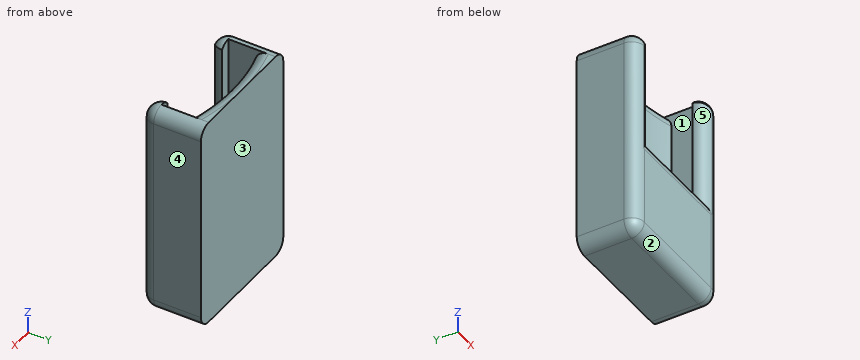
```python
from build123d import *

# Parameters (mm, degrees)
F0_W         = 53
F0_H         = 23.8
F0_W_2       = 43
F0_H_2       = 13.8
F1_DEPTH     = 80
F2_DEPTH     = 5
F3_W         = 35
F3_H         = 44
F4_DEPTH     = 25
F5_T1_DEPTH  = 78
F5_T3_DEPTH  = 110
F5_T5_DEPTH  = 35
F5_T7_DEPTH  = 56.5
F5_T13_DEPTH = 69
F5_T17_DEPTH = 47.5
F5_T24_DEPTH = 47.5
F5_T28_DEPTH = 69
F6_T1_DEPTH  = 31.3
F6_S5_W      = 5
F6_S5_H      = 5
F6_T6_DEPTH  = 5
F6_S11_W     = 5
F6_S11_H     = 5
F6_T12_DEPTH = 5
F7_R         = 4.99999
F9_DEPTH     = 80
F10_T4_ANGLE = 50.0121835392


# Not quite as in the source:
# - a fillet or chamfer that OpenCascade refuses, or shapes differently, is made with other operations: its cross-section is extruded or revolved along the edge and cut away or added
# - a fillet or chamfer is up to 0.001 mm smaller than in the source, because OpenCascade refuses the exact size


with BuildPart() as f1:
    # F0 (on Top) → F1 (new body)
    with BuildSketch(Plane.XY):
        with Locations((-2.25, 0.0045082584)):
            Rectangle(F0_W, F0_H)
        with Locations((-2.25, 0.0045082584)):
            Rectangle(F0_W_2, F0_H_2, mode=Mode.SUBTRACT)
    extrude(amount=F1_DEPTH)

    # F0 (on Top) → F2 (join)
    with BuildSketch(Plane.XY):
        with Locations((-2.25, 0.0045082584)):
            Rectangle(F0_W, F0_H)
        with Locations((-2.25, 0.0045082584)):
            Rectangle(F0_W_2, F0_H_2, mode=Mode.SUBTRACT)
        with Locations((-2.25, 0.0045082584)):
            Rectangle(F0_W_2, F0_H_2)
    extrude(amount=-F2_DEPTH)

    # F3 (on face) → F4 (cut)
    with BuildSketch(Plane(origin=(0, -6.8954917416, 0), x_dir=(-1, 0, 0), z_dir=(0, 1, 0))):
        with Locations((2.25, 58)):
            Rectangle(F3_W, F3_H)
    extrude(amount=-F4_DEPTH, mode=Mode.SUBTRACT)

    # F5: fillet of radius 5 on 6 edges, made by hand

    # F5_s2 → F5_t1 (cut)
    with BuildSketch(Plane.YZ.offset(-41.25)):
        with BuildLine():
            ThreePointArc((-11.8954917416, 0), (-10.4310256475, -3.5355339059), (-6.8954917416, -5))
            Line((-6.8954917416, -5), (-11.8954917416, -5))
            Line((-11.8954917416, -5), (-11.8954917416, 0))
        make_face()
    extrude(amount=F5_T1_DEPTH, mode=Mode.SUBTRACT)

    # F5_s4 → F5_t3 (cut)
    with BuildSketch(Plane.XY.offset(-17.5)):
        with BuildLine():
            ThreePointArc((-23.75, -11.8954917416), (-27.2855339059, -10.4310256475), (-28.75, -6.8954917416))
            Line((-28.75, -6.8954917416), (-28.75, -11.8954917416))
            Line((-28.75, -11.8954917416), (-23.75, -11.8954917416))
        make_face()
        with BuildLine():
            ThreePointArc((24.25, -6.8954917416), (22.7855339059, -10.4310256475), (19.25, -11.8954917416))
            Line((19.25, -11.8954917416), (24.25, -11.8954917416))
            Line((24.25, -11.8954917416), (24.25, -6.8954917416))
        make_face()
    extrude(amount=F5_T3_DEPTH, mode=Mode.SUBTRACT)

    # F5_s6 → F5_t5 (cut)
    with BuildSketch(Plane.YZ.offset(-19.75)):
        with BuildLine():
            ThreePointArc((-11.8954917416, 31), (-10.4310256475, 34.5355339059), (-6.8954917416, 36))
            Line((-6.8954917416, 36), (-11.8954917416, 36))
            Line((-11.8954917416, 36), (-11.8954917416, 31))
        make_face()
    extrude(amount=F5_T5_DEPTH, mode=Mode.SUBTRACT)

    # F5_s8 → F5_t7 (cut)
    with BuildSketch(Plane.XY.offset(36)):
        with BuildLine():
            ThreePointArc((-24.75, -11.8954917416), (-21.2144660941, -10.4310256475), (-19.75, -6.8954917416))
            Line((-19.75, -6.8954917416), (-19.75, -11.8954917416))
            Line((-19.75, -11.8954917416), (-24.75, -11.8954917416))
        make_face()
        with BuildLine():
            ThreePointArc((20.25, -11.8954917416), (16.7144660941, -10.4310256475), (15.25, -6.8954917416))
            Line((15.25, -6.8954917416), (15.25, -11.8954917416))
            Line((15.25, -11.8954917416), (20.25, -11.8954917416))
        make_face()
    extrude(amount=F5_T7_DEPTH, mode=Mode.SUBTRACT)


with BuildPart() as f5_tool11:
    # F5_s12 → F5_t13 (new body)
    with BuildSketch(Plane.XY.offset(92.5)):
        with BuildLine():
            ThreePointArc((20.25, -11.8954917416), (16.7144660941, -10.4310256475), (15.25, -6.8954917416))
            Line((15.25, -6.8954917416), (15.25, -11.8954917416))
            Line((15.25, -11.8954917416), (20.25, -11.8954917416))
        make_face()
    extrude(amount=-F5_T13_DEPTH)

    split(bisect_by=Plane.XY.offset(36), keep=Keep.BOTTOM)


with BuildPart() as f5_tool15:
    # F5_s16 → F5_t17 (new body)
    with BuildSketch(Plane.YZ.offset(27.75)):
        with BuildLine():
            ThreePointArc((-11.8954917416, 31), (-10.4310256475, 34.5355339059), (-6.8954917416, 36))
            Line((-6.8954917416, 36), (-11.8954917416, 36))
            Line((-11.8954917416, 36), (-11.8954917416, 31))
        make_face()
    extrude(amount=-F5_T17_DEPTH)

    split(bisect_by=Plane.YZ.offset(15.25), keep=Keep.TOP)


with BuildPart() as f5_tool11_1:
    add(f5_tool11.part)

    # F5_t19: intersect F5_tool15
    add(f5_tool15.part, mode=Mode.INTERSECT)


with BuildPart() as f1_1:
    add(f1.part)

    # F5_t9: cut F5_tool11
    add(f5_tool11_1.part, mode=Mode.SUBTRACT)


with BuildPart() as f5_tool22:
    # F5_s23 → F5_t24 (new body)
    with BuildSketch(Plane.YZ.offset(15.25)):
        with BuildLine():
            ThreePointArc((-11.8954917416, 31), (-10.4310256475, 34.5355339059), (-6.8954917416, 36))
            Line((-6.8954917416, 36), (-11.8954917416, 36))
            Line((-11.8954917416, 36), (-11.8954917416, 31))
        make_face()
    extrude(amount=-F5_T24_DEPTH)

    split(bisect_by=Plane.YZ.offset(-19.75), keep=Keep.BOTTOM)


with BuildPart() as f5_tool26:
    # F5_s27 → F5_t28 (new body)
    with BuildSketch(Plane.XY.offset(23.5)):
        with BuildLine():
            ThreePointArc((-24.75, -11.8954917416), (-21.2144660941, -10.4310256475), (-19.75, -6.8954917416))
            Line((-19.75, -6.8954917416), (-19.75, -11.8954917416))
            Line((-19.75, -11.8954917416), (-24.75, -11.8954917416))
        make_face()
    extrude(amount=F5_T28_DEPTH)

    split(bisect_by=Plane.XY.offset(36), keep=Keep.BOTTOM)


with BuildPart() as f5_tool22_1:
    add(f5_tool22.part)

    # F5_t30: intersect F5_tool26
    add(f5_tool26.part, mode=Mode.INTERSECT)


with BuildPart() as f1_2:
    add(f1_1.part)

    # F5_t20: cut F5_tool22
    add(f5_tool22_1.part, mode=Mode.SUBTRACT)

    # F6: fillet of radius 5 on 2 edges, made by hand

    # F6_s2 → F6_t1 (cut)
    with BuildSketch(Plane.XZ.offset(-24.4045082584)):
        with BuildLine():
            ThreePointArc((24.25, 0), (22.7855339059, -3.5355339059), (19.25, -5))
            Line((19.25, -5), (24.25, -5))
            Line((24.25, -5), (24.25, 0))
        make_face()
        with BuildLine():
            ThreePointArc((-28.75, 0), (-27.2855339059, -3.5355339059), (-23.75, -5))
            Line((-23.75, -5), (-28.75, -5))
            Line((-28.75, -5), (-28.75, 0))
        make_face()
    extrude(amount=F6_T1_DEPTH, mode=Mode.SUBTRACT)


with BuildPart() as f6_tool4:
    # F6_s5 → F6_t6 (new body)
    with BuildSketch(Plane.YZ.offset(-23.75)):
        with Locations((-9.3954917416, -2.5)):
            Rectangle(F6_S5_W, F6_S5_H)
    extrude(amount=-F6_T6_DEPTH)

    # F6_s7 → F6_t8 (revolve, cut)
    with BuildSketch(Plane(origin=(-23.75, -6.8954917416, 0), x_dir=(0, 0.7071067812, 0.7071067812), z_dir=(0, -0.7071067812, 0.7071067812))):
        with BuildLine():
            ThreePointArc((0, -5), (5, 0), (0, 5))
            Line((0, 5), (0, -5))
        make_face()
    revolve(axis=Axis((-23.75, -6.8954917416, 0), (-1, 0, 0)), mode=Mode.SUBTRACT)


with BuildPart() as f1_3:
    add(f1_2.part)

    # F6_t3: cut F6_tool4
    add(f6_tool4.part, mode=Mode.SUBTRACT)


with BuildPart() as f6_tool10:
    # F6_s11 → F6_t12 (new body)
    with BuildSketch(Plane.YZ.offset(19.25)):
        with Locations((-9.3954917416, -2.5)):
            Rectangle(F6_S11_W, F6_S11_H)
    extrude(amount=F6_T12_DEPTH)

    # F6_s13 → F6_t14 (revolve, cut)
    with BuildSketch(Plane(origin=(19.25, -6.8954917416, 0), x_dir=(0, 0.7071067812, 0.7071067812), z_dir=(0, 0.7071067812, -0.7071067812))):
        with BuildLine():
            ThreePointArc((0, -5), (5, 0), (0, 5))
            Line((0, 5), (0, -5))
        make_face()
    revolve(axis=Axis((19.25, -6.8954917416, 0), (1, 0, 0)), mode=Mode.SUBTRACT)


with BuildPart() as f1_4:
    add(f1_3.part)

    # F6_t9: cut F6_tool10
    add(f6_tool10.part, mode=Mode.SUBTRACT)

    # F7 (radius 5 in the source; OpenCascade refuses exactly that, so slightly less here)
    f7_edges = [f1_4.edges().sort_by_distance(p)[0] for p in [
        (22.958099, -10.249594, 80),
        (-28.75, 2.504508, 80),
    ]]
    fillet(f7_edges, radius=F7_R)

    # F8 (on face) → F9 (join)
    with BuildSketch(Plane.XY):
        with BuildLine():
            ThreePointArc((-2.25, 6.9045082584), (8.604146673, 6.1508927486), (19.25, 3.9045082584))
            Line((19.25, 3.9045082584), (19.25, 6.9045082584))
            Line((19.25, 6.9045082584), (-2.25, 6.9045082584))
        make_face()
        with BuildLine():
            ThreePointArc((-23.75, 3.9045082584), (-13.104146673, 6.1508927486), (-2.25, 6.9045082584))
            Line((-2.25, 6.9045082584), (-23.75, 6.9045082584))
            Line((-23.75, 6.9045082584), (-23.75, 3.9045082584))
        make_face()
    extrude(amount=F9_DEPTH)

    # F10: fillet of radius 5 on 1 edges, made by hand


with BuildPart() as f10_tool2:
    # F10_s3 → F10_t4 (revolve)
    with BuildSketch(Plane(origin=(-29.2914715623, -13.6626291921, 0), x_dir=(0, 0, 1), z_dir=(-0.9062628485, -0.4227146193, 0))):
        with BuildLine():
            ThreePointArc((75, 14.5706793202), (78.5355339059, 16.0351454142), (80, 19.5706793202))
            Line((80, 19.5706793202), (80, 14.5706793202))
            Line((80, 14.5706793202), (75, 14.5706793202))
        make_face()
    revolve(axis=Axis((-2.25, -71.6371584083, 80), (0, 0, -1)), revolution_arc=F10_T4_ANGLE)

    split(bisect_by=Plane.YZ.offset(19.25), keep=Keep.BOTTOM)

    split(bisect_by=Plane.YZ.offset(-23.75), keep=Keep.TOP)


with BuildPart() as f1_5:
    add(f1_4.part)

    # F10_t1: cut F10_tool2
    add(f10_tool2.part, mode=Mode.SUBTRACT)


solid = f1_5.part
```
The model under review builds one solid part; all positions refer to its coordinate system, in mm. Face numbers are marked on the shaded views. A direction names the side the tool comes from. Give positions to 0.01 mm unless a question says otherwise; leave off trailing zeros. Write each loop counter-clockwise with the first axis right and the second up, starting at its lowest first coordinate (ties: lowest second). Pieces come first, ordered by that corner, then holes. Notation, with made-up numbers: M 41.5,6 L 53.5,6 A16 ccw 53.5,34 Z; hole C -27.5,-5.75 d4. An arc over 180 degrees is marked long. Answer in a Markdown table with one row per item.
Item 1: For P1, Ø1.5, axis at x = -10.5, y = 3.5, coming from the +Z side; P2, Ø6, axis at y = -9, z = 25.5, coming from the -X side, all flat-tipped, find the tip position at first contact; note any pin that passes through.
Check sheet entries:
| item | result |
|---|---|
| P1 | z = 0 |
| P2 | x = -28.75 |
Item 2: Add section C-C on z = 66. Give the boundary of the cut face in (x, y), plus the area to 3 significant figures.
Check sheet entries:
| item | result |
|---|---|
| outline | M -28.75,-6.9 A5 ccw -24.25,-11.87 A5 ccw -19.75,-6.9 L -23.75,-6.9 L -23.75,3.9 A78.54 cw 19.25,3.9 L 19.25,-6.9 L 15.25,-6.9 A5 ccw 19.75,-11.87 A5 ccw 24.25,-6.9 L 24.25,11.9 L -28.75,11.9 Z |
| area | 514 mm2 |
Item 3: Tool access review of the marked faces 1 and 2: name each direction out of +Z, -Z, +X, -X, +Y, -Y from which nothing blocks a thin tool from reaching the whole face with its end or side.
Check sheet entries:
| item | result |
|---|---|
| face 1 | +Z |
| face 2 | -Z, +X, -X, -Y |
Item 4: For line 1 along X through (y, z) = (-1, 40); line 2 along Z through (x, y) = (-15, -0.75); line 3 along X through (y, z) = (-9.75, 43), list the stretches that pass through material, from the lowest coordinate up.
Check sheet entries:
| item | result |
|---|---|
| line 1 | -28.75 to -23.75, 19.25 to 24.25 |
| line 2 | -5 to 0 |
| line 3 | -27.86 to -20.64, 16.14 to 23.36 |
Item 5: Add section B-B on z = 19.5. Give the boundary of the cut face in (x, y).
Check sheet entries:
| item | result |
|---|---|
| outline | M -28.75,-6.9 A5 ccw -23.75,-11.9 L 19.25,-11.9 A5 ccw 24.25,-6.9 L 24.25,11.9 L -28.75,11.9 Z; hole M -23.75,-6.9 L 19.25,-6.9 L 19.25,3.9 A78.54 ccw -23.75,3.9 Z |
Item 6: Draft analysis for pull direction X (two halves, no side actions). For the marked faces 3, 4 and 5, state which applies: +X half, -X half, draft (parallel to the pull), parting line (faces both ways), or undercut.
Check sheet entries:
| item | result |
|---|---|
| face 3 | draft |
| face 4 | +X half |
| face 5 | undercut |
